Source: CAD feature listing. Evaluate the final solid. Frame: model axes, mm. A direction names the side the tool comes from. Give positions to 0.01 mm unless a question says otherwise; leave off trailing zeros. Order: outer loops, then holes, each group sorted by start corner. A loop starts at its lowest first (then second) coordinate and runs counter-clockwise, first axis right, second up. Notation, with made-up numbers: (89.5, 63) -> (98.5, 63) arc R14 ccw to (98.5, 90) -> close; hole circle Ø7 at (25, 89.5). An arc over 180 degrees is marked (long way). Answer in a Markdown table with one row per item.
```python
from build123d import *

# Parameters (mm, degrees)
SKETCH2_W               = 8
SKETCH2_H               = 20
SKETCH2_W_2             = 11.75
SKETCH2_H_2             = 12.66
BOSS_EXTRUDE1_DEPTH     = 5
SKETCH3_W               = 13.1
SKETCH3_H               = 7
BOSS_EXTRUDE2_DEPTH     = 28
SKETCH4_W               = 5.75
SKETCH4_H               = 12.66
CUT_EXTRUDE1_DEPTH      = 62.587336361
SKETCH5_R               = 2
CUT_EXTRUDE2_DEPTH      = 61.902073035
SKETCH6_R               = 2
CUT_EXTRUDE3_DEPTH      = 60.059292241
SKETCH7_W               = 7
SKETCH7_H               = 28
BOSS_EXTRUDE3_DEPTH     = 19.4
SKETCH8_W               = 27
SKETCH8_H               = 33
BOSS_EXTRUDE4_DEPTH     = 2
SKETCH9_W               = 27
SKETCH9_H               = 33
BOSS_EXTRUDE5_DEPTH     = 2
CUT_EXTRUDE4_DEPTH      = 68.4388612
CUT_EXTRUDE4_DEPTH_BACK = 68.4388612
SKETCH11_W              = 12.66
SKETCH11_H              = 33
CUT_EXTRUDE5_DEPTH      = 48.572287101
SKETCH12_R              = 2
CUT_EXTRUDE6_DEPTH      = 61.695963622
SKETCH13_R              = 4
SKETCH13_R_2            = 2
CUT_EXTRUDE7_DEPTH      = 2.8


with BuildPart() as part:
    # Sketch2 → Boss-Extrude1 (new body)
    with BuildSketch(Plane(origin=(0, 0, 0), x_dir=(1, 0, 0), z_dir=(0, 1, 0))):
        with Locations((-4, 10)):
            Rectangle(SKETCH2_W, SKETCH2_H)
        Polygon((40, 0), (0, 0), (-8, 0), (-8, -7), (3.75, -7), (16.85, -7), (28.6, -7), (48, -7), (48, 0), align=None)
        with Locations((-2.125, -13.33)):
            Rectangle(SKETCH2_W_2, SKETCH2_H_2)
        with Locations((22.725, -13.33)):
            Rectangle(SKETCH2_W_2, SKETCH2_H_2)
        with Locations((44, 10)):
            Rectangle(SKETCH2_W, SKETCH2_H)
    extrude(amount=BOSS_EXTRUDE1_DEPTH)

    # Sketch3 → Boss-Extrude2 (add)
    with BuildSketch(Plane.XZ):
        Polygon((3.75, 19.66), (-8, 19.66), (-8, 0), (0, 0), (3.75, 0), (3.75, 7), align=None)
        with Locations((10.3, 3.5)):
            Rectangle(SKETCH3_W, SKETCH3_H)
        Polygon((16.85, 19.66), (16.85, 7), (16.85, 0), (28.6, 0), (28.6, 7), (28.6, 19.66), align=None)
    extrude(amount=BOSS_EXTRUDE2_DEPTH)

    # Sketch4 → Cut-Extrude1 (cut, through all)
    with BuildSketch(Plane.XZ.offset(28)):
        with Locations((-5.125, 13.33)):
            Rectangle(SKETCH4_W, SKETCH4_H)
        with Locations((25.725, 13.33)):
            Rectangle(SKETCH4_W, SKETCH4_H)
    extrude(amount=-CUT_EXTRUDE1_DEPTH, mode=Mode.SUBTRACT)

    # Sketch5 → Cut-Extrude2 (cut, through all)
    with BuildSketch(Plane.ZY.offset(2.25)):
        with Locations((13.33, -2)):
            Circle(SKETCH5_R)
        with Locations((13.33, -21)):
            Circle(SKETCH5_R)
        with Locations((13.33, -11.5)):
            Circle(SKETCH5_R)
    extrude(amount=-CUT_EXTRUDE2_DEPTH, mode=Mode.SUBTRACT)

    # Sketch6 → Cut-Extrude3 (cut, through all)
    with BuildSketch(Plane.XZ):
        with Locations(Location((43.95, -5, 0), (0, 0, 270))):
            Circle(SKETCH6_R)
        with Locations(Location((43.95, -15, 0), (0, 0, 270))):
            Circle(SKETCH6_R)
        with Locations(Location((-3.95, -5, 0), (0, 0, 270))):
            Circle(SKETCH6_R)
        with Locations(Location((-3.95, -15, 0), (0, 0, 270))):
            Circle(SKETCH6_R)
    extrude(amount=-CUT_EXTRUDE3_DEPTH, mode=Mode.SUBTRACT)

    # Sketch7 → Boss-Extrude3 (add)
    with BuildSketch(Plane(origin=(28.6, 0, 0), x_dir=(0, 0, -1), z_dir=(1, 0, 0))):
        with Locations((-3.5, -14)):
            Rectangle(SKETCH7_W, SKETCH7_H)
    extrude(amount=BOSS_EXTRUDE3_DEPTH)

    # Sketch8 → Boss-Extrude4 (add)
    with BuildSketch(Plane(origin=(48, 0, 0), x_dir=(0, 0, -1), z_dir=(1, 0, 0))):
        with Locations((6.5, -11.5)):
            Rectangle(SKETCH8_W, SKETCH8_H)
    extrude(amount=BOSS_EXTRUDE4_DEPTH)

    # Sketch9 → Boss-Extrude5 (add)
    with BuildSketch(Plane.ZY.offset(8)):
        with Locations((-6.5, -11.5)):
            Rectangle(SKETCH9_W, SKETCH9_H)
    extrude(amount=BOSS_EXTRUDE5_DEPTH)

    # Sketch10 → Cut-Extrude4 (cut, two sides: drawn at the far end of the back side and taken through both)
    with BuildSketch(Plane.ZY.offset(-48).offset(-CUT_EXTRUDE4_DEPTH_BACK)):
        Polygon((-20, 0), (0, -28), (-20, -28), align=None)
    extrude(amount=CUT_EXTRUDE4_DEPTH + CUT_EXTRUDE4_DEPTH_BACK, mode=Mode.SUBTRACT)

    # Sketch11 → Cut-Extrude5 (cut, through all)
    with BuildSketch(Plane(origin=(22.85, 0, 0), x_dir=(0, 0, -1), z_dir=(1, 0, 0))):
        with Locations((-13.33, -11.5)):
            Rectangle(SKETCH11_W, SKETCH11_H)
    extrude(amount=-CUT_EXTRUDE5_DEPTH, mode=Mode.SUBTRACT)

    # Sketch12 → Cut-Extrude6 (cut, through all)
    with BuildSketch(Plane(origin=(0, 0, 0), x_dir=(-1, 0, 0), z_dir=(0, 0, -1))):
        with Locations((-43, -5)):
            Circle(SKETCH12_R)
        with Locations((3, -5)):
            Circle(SKETCH12_R)
        with Locations((3, -21)):
            Circle(SKETCH12_R)
        with Locations((-43, -21)):
            Circle(SKETCH12_R)
        with Locations((-20, -5)):
            Circle(SKETCH12_R)
        with Locations((-20, -21)):
            Circle(SKETCH12_R)
    extrude(amount=-CUT_EXTRUDE6_DEPTH, mode=Mode.SUBTRACT)

    # Sketch13 → Cut-Extrude7 (cut)
    # profile 1 of 6: a face of its own
    with BuildSketch(Plane(origin=(0, 0, 0), x_dir=(-1, 0, 0), z_dir=(0, 0, -1))):
        with Locations((3, -5)):
            Circle(SKETCH13_R)
        with Locations((3, -5)):
            Circle(SKETCH13_R_2, mode=Mode.SUBTRACT)
    # profile 2 of 6: a face of its own
    with BuildSketch(Plane(origin=(0, 0, 0), x_dir=(-1, 0, 0), z_dir=(0, 0, -1))):
        with Locations((-43, -5)):
            Circle(SKETCH13_R)
        with Locations((-43, -5)):
            Circle(SKETCH13_R_2, mode=Mode.SUBTRACT)
    # profile 3 of 6: a face of its own
    with BuildSketch(Plane(origin=(0, 0, 0), x_dir=(-1, 0, 0), z_dir=(0, 0, -1))):
        with Locations((3, -21)):
            Circle(SKETCH13_R)
    # profile 4 of 6: a face of its own
    with BuildSketch(Plane(origin=(0, 0, 0), x_dir=(-1, 0, 0), z_dir=(0, 0, -1))):
        with Locations((-43, -21)):
            Circle(SKETCH13_R)
    # profile 5 of 6: a face of its own
    with BuildSketch(Plane(origin=(0, 0, 0), x_dir=(-1, 0, 0), z_dir=(0, 0, -1))):
        with Locations((-20, -21)):
            Circle(SKETCH13_R)
    # profile 6 of 6: a face of its own
    with BuildSketch(Plane(origin=(0, 0, 0), x_dir=(-1, 0, 0), z_dir=(0, 0, -1))):
        with Locations((-20, -5)):
            Circle(SKETCH13_R)
    extrude(amount=-CUT_EXTRUDE7_DEPTH, mode=Mode.SUBTRACT)


solid = part.part
```
(1) Pull-direction query (X, two-part tool) for faces 5 (the flat face through (42, -3, 2.8)), 6 (the flat face through (-5, 2, -20)); classes: +X half, -X half, draft (parallel to the pull), parting line (faces both ways), or undercut.
A:
| item | result |
|---|---|
| face 5 | undercut |
| face 6 | draft |
(2) Section query D-D (y = -5). Give the number of separate pieces and of enclosed holes in the cut face, plus the area to 3 significant figures.
A:
| item | result |
|---|---|
| separate pieces | 4 |
| enclosed holes | 0 |
| area | 368 mm^2 |
(3) Access query for faces 1 (the cylindrical face through (-3, -19, 5)), 2 (the flat face through (0, 2, -10)), 3 (the flat face through (44, 0, -10)), 4 (the cylindrical face through (-5.15, -17.627, 1.38)). Directions: +Z, -Z, +X, -X, +Y, -Y. A direction counts if a zero-diameter tool reaches every point of the face in a straight line with its end or side. Return the directions, or none.
A:
| item | result |
|---|---|
| face 1 | +Z, -Z |
| face 2 | -Z, +Y, -Y |
| face 3 | -Z, -Y |
| face 4 | -Z |
(4) Section query C-C (x = 20). Return the cut outline in (y, z), plus the area to 3 significant figures.
A:
| item | result |
|---|---|
| outline | (-28, 0) -> (-25, 0) -> (-25, 2.8) -> (-23, 2.8) -> (-23, 7) -> (-28, 7) -> close; (-19, 2.8) -> (-17, 2.8) -> (-17, 0) -> (-9, 0) -> (-9, 2.8) -> (-7, 2.8) -> (-7, 7) -> (-19, 7) -> close; (-3, 2.8) -> (-1, 2.8) -> (-1, 0) -> (5, 0) -> (5, 7) -> (-3, 7) -> close |
| area | 153 mm^2 |
(5) Ray query, probe 1 along Y at (x, z) = (43, 0.85); probe 2 along Y at (x, z) = (20, 4.1); probe 3 along X at (y, z) = (-7, 2.75). Return the intervals inside material, ascending.
A:
| item | result |
|---|---|
| probe 1 | y = -28 to -25, -17 to -9, -1 to 5 |
| probe 2 | y = -28 to -23, -19 to -7, -3 to 5 |
| probe 3 | x = -10 to -6.46, 0.46 to 16.54, 23.46 to 39.54, 46.46 to 50 |
(6) Section query A-A (z = -1.5). Return the cut outline in (x, y).
A:
| item | result |
|---|---|
| outline | (-10, -25.9) -> (-8, -25.9) -> (-8, 0) -> (0, 0) -> (0, 5) -> (-10, 5) -> close; (40, 0) -> (48, 0) -> (48, -25.9) -> (50, -25.9) -> (50, 5) -> (40, 5) -> close |
(7) Section query B-B (z = 5). Return the cut outline in (x, y).
A:
| item | result |
|---|---|
| outline | (-10, -28) -> (50, -28) -> (50, 5) -> (-10, 5) -> close; hole circle Ø4 at (-3, -21); hole circle Ø4 at (-3, -5); hole circle Ø4 at (20, -21); hole circle Ø4 at (20, -5); hole circle Ø4 at (43, -21); hole circle Ø4 at (43, -5) |
(8) First-contact query: pin 1 Ø2.5 at (x, y) = (19.5, -5.5) entering from -Z; pin 2 Ø1 at (x, y) = (15.5, -13) entering from -Z; pin 3 Ø4.5 at (x, y) = (43, -21) entering from -Z; pin 4 Ø4 at (x, z) = (42.5, -11.5) entering from -Y. Flat tips, straight axial feed; report the tip coordinate or a pass-through.
A:
| item | result |
|---|---|
| pin 1 | passes through |
| pin 2 | stops at z = 0 |
| pin 3 | stops at z = 2.8 |
| pin 4 | stops at y = 0 |
